Input: part model. Units: mm. Frame: model coordinates. Face numbers are marked on the shaded views. A direction names the side the tool comes from. Coordinates: 2 decimals unless noted, no trailing zeros. Write each loop counter-clockwise with the first axis right and the second up, starting at its lowest first coordinate (ties: lowest second). Pieces come first, ordered by that corner, then holes. Notation, with made-up numbers: M -32,67 L 12,67 A10 ccw 12,86 Z; hole C 52,16.5 d8. An arc over 180 degrees is marked long. Write each question's results on one line, items separated by ' | '. Start each with the question number.
1. Section query C-C, the plane y = 6.75. Output: boundary loops of the cut face in (x, z).
2. Set-up query: the marked faces 5, 6, 7 and 8. Return all of +Z, -Z, +X, -X, +Y, -Y with unobstructed straight access to the full face (end or side cutting, diameter ignored); none if empty.
3. Pull-direction query (Y, two-part tool) for the marked faces 1, 2, 3 and 4; classes: +Y half, -Y half, draft (parallel to the pull), parting line (faces both ways), or undercut.
4. Section query B-B, the plane z = 14.25. Output: boundary loops of the cut face in (x, y), and give its area (3 significant figures).
5. Ray query, probe 1 along X at (y, z) = (7.5, 14.5); probe 2 along X at (y, z) = (5.25, 3.5); probe 3 along Y at (x, z) = (-6.5, 16). Return the intervals inside material, ascending.
6. Section query A-A, the plane x = -4.5. Output: boundary loops of the cut face in (y, z).
7. First-contact query: pin 1 (8 mm diameter, centred on x = 8, z = 4, fed in from +Y); pin 2 (1.5 mm diameter, centred on x = 4, z = 11, fed in from +Y); pin 3 (1.5 mm diameter, centred on x = -4.5, z = 12, fed in from +Y). Flat tips, straight axial feed; report the tip coordinate or a pass-through.
8. Section query D-D, the plane x = -8.25. Output: boundary loops of the cut face in (y, z), and give its area (3 significant figures).
Autodesk Inventor part; units mm, degrees
ref_plane "Work Plane2" through (0, 0, 10) normal (0, 0, 1) x (1, 0, 0)
ref_plane "Work Plane8" through (0, 0, 0) normal (0.9009689, 0.4338837, 0) x (0, 0, 1)
ref_plane "Work Plane9" through (0, 0, 0) normal (1, 0, 0) x (0, 1, 0)
sketch "Sketch1" plane through (0, 0, 0) normal (0, 0, 1) x (1, 0, 0)
  circle A0 centre (0, 0) radius 10.1879
  dimension "d0" = 20.3758
extrude "Extrusion1" add sketch "Sketch1" along normal blind 20
ref_plane "Work Plane2" through (0, 0, 10) normal (0, 0, 1) x (1, 0, 0)
sketch "Sketch2" plane through (0, 0, 0) normal (0, 0, -1) x (-1, 0, 0)
  circle A0 centre (0, 0) radius 10.1879
  circle A1 centre (0, 0) radius 7.147
  dimension "d3" = 14.2941
surface extrude "Pitch Diameter" sketch "Sketch2" against normal through all shown no curves A1
ref_plane "Work Plane8" through (0, 0, 0) normal (0.9009689, 0.4338837, 0) x (0, 0, 1)
ref_plane "Work Plane9" through (0, 0, 0) normal (1, 0, 0) x (0, 1, 0)
spur gear teeth "Spur Gear" teeth 7 pitch diameter 14 tip diameter 20.3758 root diameter 11.6787 face width 20 start plane through (0, 0, 0) normal (0, 0, -1) x (-1, 0, 0)
equation "\"d0\" = da_da"
equation "\"d1\" = da_b"
equation "\"d3\" = da_dw"
equation "\"d16\" = da_aw"
equation "\"d43\" = da_aw"
equation "\"d46\" = da_aw"
properties part number "Spur Gear1" material "Steel"
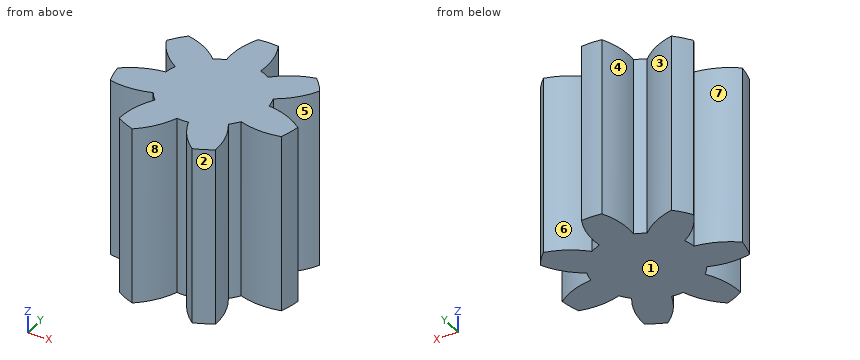
Answer:
1) outline: M -7.63,0 L -5.77,0 L -5.77,20 L -7.63,20 Z; M -1.98,0 L 1.98,0 L 1.98,20 L -1.98,20 Z; M 5.77,0 L 7.63,0 L 7.63,20 L 5.77,20 Z
2) face 5: +Z, -Z, +X | face 6: +Z, -Z, +Y | face 7: +Z, -Z, -X | face 8: +Z, -Z, -Y
3) face 1: draft | face 2: -Y half | face 3: +Y half | face 4: undercut
4) outline: M -10.12,-1.14 A10.19 ccw -9.62,-3.36 A8.25 ccw -4.94,-3.11 A5.84 ccw -4.13,-4.13 A8.25 ccw -5.42,-8.63 A10.19 ccw -3.36,-9.62 A8.25 ccw -0.65,-5.8 A5.84 ccw 0.65,-5.8 A8.25 ccw 3.36,-9.62 A10.19 ccw 5.42,-8.63 A8.25 ccw 4.13,-4.13 A5.84 ccw 4.94,-3.11 A8.25 ccw 9.62,-3.36 A10.19 ccw 10.12,-1.14 A8.25 ccw 5.8,0.65 A5.84 ccw 5.51,1.93 A8.25 ccw 8.63,5.42 A10.19 ccw 7.2,7.2 A8.25 ccw 3.11,4.94 A5.84 ccw 1.93,5.51 A8.25 ccw 1.14,10.12 A10.19 ccw -1.14,10.12 A8.25 ccw -1.93,5.51 A5.84 ccw -3.11,4.94 A8.25 ccw -7.2,7.2 A10.19 ccw -8.63,5.42 A8.25 ccw -5.51,1.93 A5.84 ccw -5.8,0.65 A8.25 ccw Z | area: 216 mm^2
5) probe 1: -1.92 to 1.92 | probe 2: -8.54 to -3.43, -2.56 to 2.56, 3.43 to 8.54 | probe 3: -3.5 to 0.55, 2.65 to 7.02
6) outline: M -9.14,0 L -4.77,0 L -4.77,20 L -9.14,20 Z; M -3.72,0 L 6.08,0 L 6.08,20 L -3.72,20 Z
7) pin 1: y = 7.2 | pin 2: y = 6.23 | pin 3: y = 6.51
8) outline: M -3.57,0 L 0,0 L 0,20 L -3.57,20 Z; M 4.71,0 L 5.98,0 L 5.98,20 L 4.71,20 Z | area: 96.7 mm^2
